from build123d import *

# Parameters (mm, degrees)
SKETCH2_W               = 12.5
SKETCH2_H               = 2
CUT_EXTRUDE1_DEPTH      = 29
CUT_EXTRUDE2_REACH      = 60.017
CUT_EXTRUDE2_END_RADIUS = 8
SKETCH4_R               = 2
SKETCH5_R               = 8
CUT_EXTRUDE3_DEPTH      = 2


with BuildPart() as part:
    # Sketch1 → Revolve1 (revolve)
    with BuildSketch(Plane.XY, mode=Mode.PRIVATE) as revolve1_sk:
        Polygon((4, 0), (4, 54), (15, 54), (15, 49), (12.5, 49), (12.5, 20), (8, 20), (8, 0), align=None)
    revolve(revolve1_sk.sketch.rotate(Axis((0, 0, 0), (0, 1, 0)), 90), axis=Axis((0, 0, 0), (0, 1, 0)))

    # Sketch2 → Cut-Extrude1 (cut)
    with BuildSketch(Plane.XZ.offset(-20)):
        with Locations((0, 11.825317547)):
            Rectangle(SKETCH2_W, SKETCH2_H)
    extrude(amount=-CUT_EXTRUDE1_DEPTH, mode=Mode.SUBTRACT)

    # Cut-Extrude2: up to this cylinder (the profile starts inside it)
    cut_extrude2_end = Plane(origin=(0, 10, 0), z_dir=(0, -1, 0)) * Cylinder(CUT_EXTRUDE2_END_RADIUS, 137.034, mode=Mode.PRIVATE)
    # Sketch4 → Cut-Extrude2 (cut, up to the surface)
    with BuildSketch(Plane.XY, mode=Mode.PRIVATE) as cut_extrude2_sk1:
        with Locations(Location((0, 10, 0), (0, 0, 180))):
            Circle(SKETCH4_R)
    cut_extrude2_tool1 = extrude(cut_extrude2_sk1.sketch, amount=CUT_EXTRUDE2_REACH, mode=Mode.PRIVATE) & cut_extrude2_end
    add(cut_extrude2_tool1.solids().sort_by_distance((0, 10, 0))[0], mode=Mode.SUBTRACT)

    # Sketch5 → Cut-Extrude3 (cut)
    with BuildSketch(Plane.XZ):
        with Locations(Location((0, 0, 0), (0, 0, 270))):
            Circle(SKETCH5_R)
    extrude(amount=-CUT_EXTRUDE3_DEPTH, mode=Mode.SUBTRACT)


solid = part.part
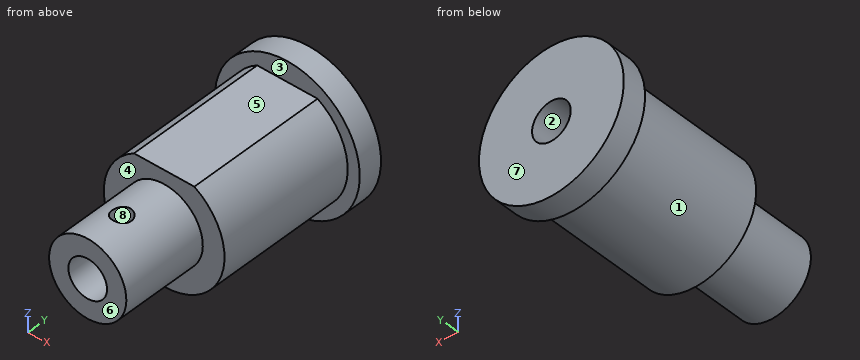
Read the model definition and answer for the solid it produces. Units are mm, in the model's axes. Face numbers are marked on the shaded views. A direction names the side the tool comes from. Coordinates: 2 decimals unless noted, no trailing zeros. Loops run counter-clockwise (first coordinate to the right, second up) from the corner with the lowest first, then second, coordinate; pieces in that order, holes last.
Q1. The mould has two halves that part along X. Classify the marked faces 1, 2 and 3: +X half, -X half, draft (parallel to the pull), parting line (faces both ways), or undercut.
Q2. The part is cut by section C-C on y = 32. Write down the section's boundary in (x, z), and give its area (3 significant figures).
Q3. The part is cut by section B-B on z = 0. Write down the section's boundary in (x, y).
Q4. The part is cut by section A-A on x = 0. Write down the section's boundary in (y, z).
Q5. Each of these flat-tipped pins is pushed along its axis until it touches: pin 1 Ø4 at (y, z) = (30.5, -8.5) entering from -X; pin 2 Ø3 at (x, y) = (-4.5, 24.5) entering from -Z; pin 3 Ø4 at (y, z) = (10.5, -6.5) entering from -X. Where does it stop, or does it pass through?
Q6. Which of the six approach directions +Z, -Z, +X, -X, +Y, -Y give full straight-line access (tool end or side, diameter ignored) to the marked faces 4, 5, 6, 7 and 8?
Q7. Consider probe 1 along X at (y, z) = (19, 0); probe 2 along Y at (x, z) = (0, 6.1); probe 3 along Y at (x, z) = (11.25, 1.25). Determine where each line is inside the solid, lowest interval first.
Q8. The part is cut by section D-D on x = -3.25. Write down the section's boundary in (y, z).
Results below:
1. face 1: parting line
1. face 2: undercut
1. face 3: draft
2. outline: (-6.25, 10.83) arc R12.5 ccw (long way) to (6.25, 10.83) - close; hole circle Ø8 at (0, 0)
2. area: 426 mm2
3. outline: (-15, 49) - (-12.5, 49) - (-12.5, 20) - (-8, 20) - (-8, 2) - (-4, 2) - (-4, 54) - (-15, 54) - close; (4, 2) - (8, 2) - (8, 20) - (12.5, 20) - (12.5, 49) - (15, 49) - (15, 54) - (4, 54) - close
4. outline: (2, -8) - (20, -8) - (20, -12.5) - (49, -12.5) - (49, -15) - (54, -15) - (54, -4) - (2, -4) - close; (2, 4) - (8, 4) - (8, 8) - (2, 8) - close; (12, 4) - (54, 4) - (54, 15) - (49, 15) - (49, 10.83) - (20, 10.83) - (20, 8) - (12, 8) - close
5. pin 1: stops at x = -10.68
5. pin 2: stops at z = -12.13
5. pin 3: stops at x = -6.61
6. face 4: -Y
6. face 5: +Z, +X, -X, -Y
6. face 6: +Z, -Z, +X, -X, -Y
6. face 7: +Z, -Z, +X, -X, +Y
6. face 8: +Z
7. probe 1: x = -8 to -4, 4 to 8
7. probe 2: y = 2 to 8, 12 to 54
7. probe 3: y = 20 to 54
8. outline: (2, -7.31) - (20, -7.31) - (20, -12.07) - (49, -12.07) - (49, -14.64) - (54, -14.64) - (54, -2.33) - (2, -2.33) - close; (2, 2.33) - (54, 2.33) - (54, 14.64) - (49, 14.64) - (49, 10.83) - (20, 10.83) - (20, 7.31) - (2, 7.31) - close
